from build123d import *

# Parameters (mm, degrees)
SKETCH_R      = 8
PAD_DEPTH     = 5
SKETCH001_R   = 10
SKETCH001_R_2 = 6
PAD001_DEPTH  = 2
PAD002_DEPTH  = 2
SKETCH003_R   = 1.65
POCKET_DEPTH  = 7.001


with BuildPart() as part:
    # Sketch → Pad (new body)
    with BuildSketch(Plane.XY):
        with BuildLine():
            ThreePointArc((-2.142857, -9.76771), (10, 0), (-2.142857, 9.76771))
            Line((-28.857143, 3.907084), (-2.142857, 9.76771))
            ThreePointArc((-28.857143, 3.907084), (-32, 0), (-28.857143, -3.907084))
            Line((-2.142857, -9.76771), (-28.857143, -3.907084))
        make_face()
        Circle(SKETCH_R, mode=Mode.SUBTRACT)
    extrude(amount=PAD_DEPTH)

    # Sketch001 (on Face7 of Pad) → Pad001 (join)
    with BuildSketch(Plane.XY.offset(5)):
        Circle(SKETCH001_R)
        Circle(SKETCH001_R_2, mode=Mode.SUBTRACT)
    extrude(amount=PAD001_DEPTH)

    # Sketch002 (on Face7 of Pad001) → Pad002 (join)
    with BuildSketch(Plane.XY.offset(5)):
        with BuildLine():
            ThreePointArc((-28.857143, 3.907084), (-32, 0), (-28.857143, -3.907084))
            Line((-28.857143, -3.907084), (-22.089875, -5.391699))
            ThreePointArc((-22.089875, -5.391699), (-20, 0), (-22.089875, 5.391699))
            Line((-28.857143, 3.907084), (-22.089875, 5.391699))
        make_face()
    extrude(amount=PAD002_DEPTH)

    # Sketch003 (on Face14 of Pad002) → Pocket (cut, through all)
    with BuildSketch(Plane.XY.offset(7)):
        with Locations((-28, 0)):
            Circle(SKETCH003_R)
    extrude(amount=-POCKET_DEPTH, mode=Mode.SUBTRACT)


solid = part.part
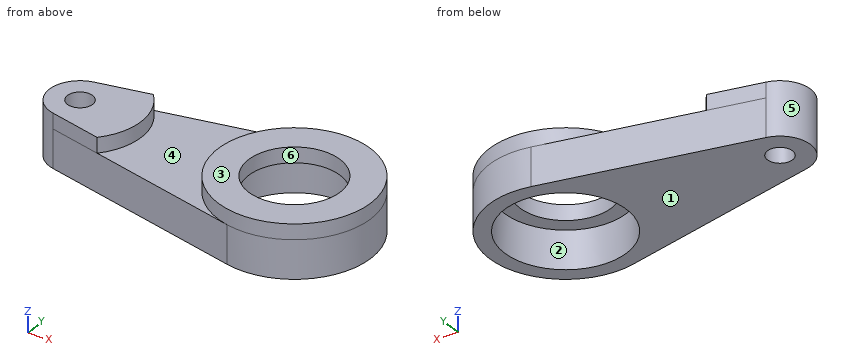
Verification items for the finished model (mm, model axes). Face numbers are marked on the shaded views. A direction names the side the tool comes from. Coordinates: 2 decimals unless noted, no trailing zeros. Order: outer loops, then holes, each group sorted by start corner. A loop starts at its lowest first (then second) coordinate and runs counter-clockwise, first axis right, second up. Notation, with made-up numbers: M -16,63 L 32,63 A14 ccw 32,77 Z; hole C 53.5,-13 d4. An arc over 180 degrees is marked long. One line per item, written item: value. Start each with the question number.
Item 1: Scan lines: probe 1 along X at (y, z) = (0.25, 4.5); probe 2 along Y at (x, z) = (0, 5.5); probe 3 along Z at (x, y) = (-20.5, -4.5). Record each from-to range of solid material in increasing order.
Item 2: Mould release check, pull along X, two halves, no side actions. Record for the marked faces 3, 4, 5 and 6: released by +X, released by -X, zero draft, split by the parting line, or undercut.
Item 3: Sectioned sample at D-D (z = 3). Enter the section's corners in (x, y), then the cut area to 3 significant figures.
Item 4: Sectioned sample at C-C (y = 0). Enter the section's corners in (x, z), then the cut area to 3 significant figures.
Item 5: Sectioned sample at B-B (z = 6.25). Enter the section's corners in (x, y).
Item 6: Gauge pin test, flat ends, axial feed: pin 1 (4 mm diameter, centred on x = -20.5, z = 5, fed in from -Y); pin 2 (1.5 mm diameter, centred on y = 2.5, z = 6, fed in from -X); pin 3 (1.5 mm diameter, centred on y = 6.5, z = 6, fed in from -X). Record the tip position at first contact, or that the pin passes through.
Item 7: Access from +Z, -Z, +X, -X, +Y, -Y to the whole of each face (thin tool, end or side, straight path). Record for the marked faces 1 and 2.
Item 8: Sectioned sample at A-A (x = 0). Enter the section's corners in (y, z), then the cut area to 3 significant figures.
Conclusion:
1. probe 1: x = -31.99 to -29.63, -26.37 to -8, 8 to 10
1. probe 2: y = -10 to -6, 6 to 10
1. probe 3: z = 0 to 5
2. face 3: zero draft
2. face 4: undercut
2. face 5: released by -X
2. face 6: undercut
3. outline: M -28.86,-3.91 L -2.14,-9.77 A10 ccw long -2.14,9.77 L -28.86,3.91 A4 ccw Z; hole C -28,0 d3.3; hole C 0,0 d16
3. area: 374 mm^2
4. outline: M -32,0 L -29.65,0 L -29.65,7 L -32,7 Z; M -26.35,0 L -8,0 L -8,5 L -6,5 L -6,7 L -10,7 L -10,5 L -20,5 L -20,7 L -26.35,7 Z; M 6,5 L 8,5 L 8,0 L 10,0 L 10,7 L 6,7 Z
4. area: 147 mm^2
5. outline: M -28.86,-3.91 L -22.09,-5.39 A8 ccw -22.09,5.39 L -28.86,3.91 A4 ccw Z; C 0,0 d20; hole C -28,0 d3.3; hole C 0,0 d12
6. pin 1: stops at y = -6.18
6. pin 2: stops at x = -31.6
6. pin 3: stops at x = -8.18
7. face 1: -Z, +X, -X, +Y, -Y
7. face 2: -Z
8. outline: M -10,0 L -8,0 L -8,5 L -6,5 L -6,7 L -10,7 Z; M 6,5 L 8,5 L 8,0 L 10,0 L 10,7 L 6,7 Z
8. area: 36.0 mm^2
